CAD build for the part. Positions are in the model's coordinates, mm. Coordinates: 2 decimals unless noted, no trailing zeros. Loops run counter-clockwise (first coordinate to the right, second up) from the corner with the lowest first, then second, coordinate; pieces in that order, holes last. Notation, with made-up numbers: (42.5, -13) -> (82.5, -13) arc R21 ccw to (82.5, 15) -> close; hole circle Ø11 at (39.25, 50.5). An arc over 180 degrees is marked (long way). Write item = value, one per line. Start each with the question number.
(1) Band-saw the part on C-C (x = 148.5). Write the cut outline in (y, z), and give its area (3 significant figures).
(2) Pull direction X, two halves, no side cores. Call faces 1 (the face through (246, 177, 5)), 2 (the face through (338.76, 67.95, 2.46)), 3 (the face through (67.36, 139.06, 2.46)): +X half, -X half, draft (parallel to the pull), parting line (faces both ways), or undercut.
(3) Flat gauge pins, fed straight in: P1, Ø2.5, axis at y = 247, z = 1.5, coming from the -X side; P2, Ø1.5, axis at y = 85, z = 1.5, coming from the -X side; P3, Ø1.5, axis at x = 433, z = 2.5, coming from the +Y side. Where does each tip first touch, or does it go through?
(4) Band-saw the part on D-D (z = 2.55). Count the separate pieces of the cut face and the enclosed holes in it, and give its area (3 significant figures).
(5) Drill centre lines: line 1 (Y direction, x = 91.7, z = 1.75); line 2 (Y direction, x = 275, z = 3.9); line 3 (X direction, y = 192, z = 3.4). Where is each one in solid material? Low to high. Write a range as from..to.
(6) Band-saw the part on A-A (x = 268). Write the cut outline in (y, z).
(7) Band-saw the part on B-B (y = 107.5). Write the cut outline in (x, z).
```python
from build123d import *

# Parameters (mm, degrees)
SKETCH1_R           = 2.1
SKETCH1_W           = 30
SKETCH1_H           = 5
SKETCH1_W_2         = 5
SKETCH1_H_2         = 30
BOSS_EXTRUDE1_DEPTH = 5


with BuildPart() as part:
    # Sketch1 → Boss-Extrude1 (new body)
    with BuildSketch(Plane.XY):
        with BuildLine():
            Line((175, 370.830805108), (95.700000001, 370.830805108))
            Line((95.700000001, 370.830805108), (87.2, 370.830805108))
            Line((87.2, 370.830805108), (87.2, 331.230805108))
            Line((87.2, 331.230805108), (87.2, 220.830805108))
            Line((87.2, 220.830805108), (87.2, 181.230805108))
            Line((87.2, 181.230805108), (46.963204669, 95.700000001))
            Line((46.963204669, 95.700000001), (46.963204669, 87.2))
            Line((46.963204669, 87.2), (86.563204669, 87.2))
            Line((86.563204669, 87.2), (155.557214446, 87.2))
            Line((155.557214446, 87.2), (195.157214446, 87.2))
            Line((195.157214446, 87.2), (195.157214446, 117.2))
            ThreePointArc((195.157214446, 117.2), (196.62168054, 120.735533906), (200.157214446, 122.2))
            Line((200.157214446, 122.2), (295.7, 122.2))
            ThreePointArc((295.7, 122.2), (299.235533906, 120.735533906), (300.7, 117.2))
            Line((300.7, 117.2), (300.7, 88.836795331))
            Line((300.7, 88.836795331), (300.7, 49.236795331))
            Line((300.7, 49.236795331), (309.200000001, 49.236795331))
            Line((309.200000001, 49.236795331), (369.169194892, 87.2))
            Line((369.169194892, 87.2), (408.769194892, 87.2))
            Line((408.769194892, 87.2), (450, 87.2))
            Line((450, 87.2), (450, 150))
            Line((450, 150), (420, 150))
            Line((420, 150), (420, 155))
            Line((420, 155), (450, 155))
            Line((450, 155), (450, 187))
            Line((450, 187), (445, 187))
            Line((445, 187), (445, 217))
            Line((445, 217), (450, 217))
            Line((450, 217), (450, 245))
            Line((450, 245), (420, 245))
            Line((420, 245), (420, 250))
            Line((420, 250), (370, 250))
            Line((370, 250), (370, 245))
            Line((370, 245), (340, 245))
            Line((340, 245), (340, 250))
            Line((340, 250), (290, 250))
            Line((290, 250), (290, 245))
            Line((290, 245), (260, 245))
            Line((260, 245), (260, 250))
            Line((260, 250), (210, 250))
            Line((210, 250), (210, 245))
            Line((210, 245), (180, 245))
            Line((180, 245), (180, 365.830805108))
            ThreePointArc((180, 365.830805108), (178.535533906, 369.366339014), (175, 370.830805108))
        make_face()
        with Locations((51.763204669, 91.700000001)):
            Circle(SKETCH1_R, mode=Mode.SUBTRACT)
        with Locations((81.763204669, 91.700000001)):
            Circle(SKETCH1_R, mode=Mode.SUBTRACT)
        with Locations((160.357214446, 91.700000001)):
            Circle(SKETCH1_R, mode=Mode.SUBTRACT)
        with Locations((190.357214446, 91.700000001)):
            Circle(SKETCH1_R, mode=Mode.SUBTRACT)
        with Locations((91.700000001, 186.030805108)):
            Circle(SKETCH1_R, mode=Mode.SUBTRACT)
        with Locations((195, 152.5)):
            Rectangle(SKETCH1_W, SKETCH1_H, mode=Mode.SUBTRACT)
        with Locations((177.5, 202)):
            Rectangle(SKETCH1_W_2, SKETCH1_H_2, mode=Mode.SUBTRACT)
        with Locations((305.200000001, 54.036795331)):
            Circle(SKETCH1_R, mode=Mode.SUBTRACT)
        with Locations((305.200000001, 84.036795331)):
            Circle(SKETCH1_R, mode=Mode.SUBTRACT)
        with Locations((373.969194892, 91.700000001)):
            Circle(SKETCH1_R, mode=Mode.SUBTRACT)
        with Locations((403.969194892, 91.700000001)):
            Circle(SKETCH1_R, mode=Mode.SUBTRACT)
        with Locations((275, 152.5)):
            Rectangle(SKETCH1_W, SKETCH1_H, mode=Mode.SUBTRACT)
        with Locations((355, 152.5)):
            Rectangle(SKETCH1_W, SKETCH1_H, mode=Mode.SUBTRACT)
        with Locations((91.700000001, 216.030805108)):
            Circle(SKETCH1_R, mode=Mode.SUBTRACT)
        with Locations((91.700000001, 336.030805108)):
            Circle(SKETCH1_R, mode=Mode.SUBTRACT)
        with Locations((91.700000001, 366.030805108)):
            Circle(SKETCH1_R, mode=Mode.SUBTRACT)
    extrude(amount=BOSS_EXTRUDE1_DEPTH)


solid = part.part
```
Findings below:
q1.outline = (87.2, 0) -> (370.83, 0) -> (370.83, 5) -> (87.2, 5) -> close
q1.area = 1,420 mm²
q2.face_1 = draft
q2.face_2 = +X half
q2.face_3 = -X half
q3.P1 = 87.2
q3.P2 = 300.7
q3.P3 = 245
q4.separate_pieces = 1
q4.enclosed_holes = 16
q4.area = 68,400 mm²
q5.line_1 = 87.2..183.93, 188.13..213.93, 218.13..333.93, 338.13..363.93, 368.13..370.83
q5.line_2 = 122.2..150, 155..245
q5.line_3 = 87.2..175, 180..445
q6.outline = (122.2, 0) -> (150, 0) -> (150, 5) -> (122.2, 5) -> close; (155, 0) -> (245, 0) -> (245, 5) -> (155, 5) -> close
q7.outline = (52.51, 0) -> (195.16, 0) -> (195.16, 5) -> (52.51, 5) -> close; (300.7, 0) -> (450, 0) -> (450, 5) -> (300.7, 5) -> close
